Can you work these out from the drawing? Everything is in mm from the part's minimum corner. A direction names the side the tool comes from. Give positions to 0.01 mm unless a question says otherwise; leave off trailing zeros. Loops run counter-clockwise (first coordinate to the right, second up) from the corner with the lowest first, then second, coordinate; pieces in that order, holes last. Notation, with made-up numbers: (-13, 10) - (30, 10) arc R18 cw to (30, 24) - close; hole circle Ø3 at (35, -11.5). An arc over 180 degrees is marked (long way). One line per item, written item: value. Start each with the question number.
Q1. I'm going to push flat-ended pins straight in: P1, Ø1.6, axis at y = 2.5, z = 10, coming from the -X side; P2, Ø1.6, axis at y = 4, z = 10, coming from the +X side; P3, Ø2, axis at y = 2, z = 20.5, coming from the -X side; P4, Ø5, axis at x = 11.44, z = 11.44, coming from the +Y side. Where does each tip first touch, or does it pass through?
Q2. If we mould it in two halves opening along X, with no side actions, what happens to the marked faces 3, 4 and 5? For each: released by +X, released by -X, zero draft, split by the parting line, or undercut.
Q3. I want a section at B-B (z = 9). Please give me the cut outline in (x, y).
Q4. I want a section at A-A (y = 2.2). Please give me the cut outline in (x, z) (1 decimal), then the cut area to 3 significant figures.
Q5. I want a section at D-D (z = 16). Please give me the cut outline in (x, y).
Q6. For the marked faces 1 and 2, which set-ups out of +Z, -Z, +X, -X, +Y, -Y let a thin tool reach every point of the face, with its end or its side?
Q7. I want a section at C-C (x = 9). Please give me the cut outline in (y, z).
Q8. If I drill on line 1 (Y direction, x = 18.25, z = 8); line 2 (X direction, y = 3.25, z = 11) (1 decimal); line 3 (Z direction, x = 7, y = 4) (1 decimal), over which ranges is the centre line in solid material (lowest first)? Write a range as from..to.
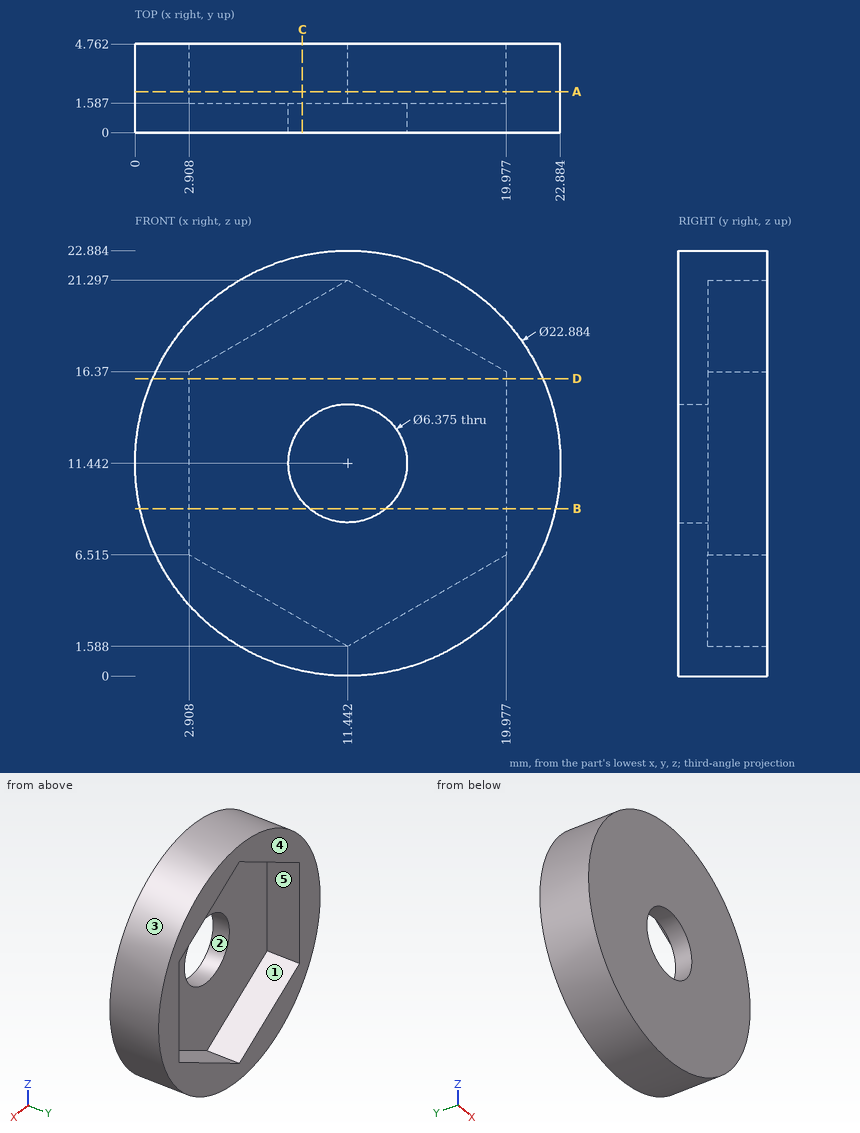
Worked answers:
1. P1: stops at x = 0.02
1. P2: stops at x = 22.87
1. P3: stops at x = 3.32
1. P4: passes through
2. face 3: split by the parting line
2. face 4: zero draft
2. face 5: undercut
3. outline: (0.26, 0) - (9.39, 0) - (9.39, 1.59) - (2.91, 1.59) - (2.91, 4.76) - (0.26, 4.76) - close; (13.49, 0) - (22.62, 0) - (22.62, 4.76) - (19.98, 4.76) - (19.98, 1.59) - (13.49, 1.59) - close
4. outline: circle Ø22.9 at (11.4, 11.4); hole (2.9, 6.5) - (11.4, 1.6) - (20, 6.5) - (20, 16.4) - (11.4, 21.3) - (2.9, 16.4) - close
4. area: 159 mm²
5. outline: (0.95, 0) - (21.94, 0) - (21.94, 4.76) - (19.98, 4.76) - (19.98, 1.59) - (2.91, 1.59) - (2.91, 4.76) - (0.95, 4.76) - close
6. face 1: +Y
6. face 2: +Y, -Y
7. outline: (0, 0.26) - (4.76, 0.26) - (4.76, 3) - (1.59, 3) - (1.59, 9.39) - (0, 9.39) - close; (0, 13.49) - (1.59, 13.49) - (1.59, 19.89) - (4.76, 19.89) - (4.76, 22.62) - (0, 22.62) - close
8. line 1: y = 0..1.59
8. line 2: x = 0..2.9, 20..22.9
8. line 3: z = 0.9..4.2, 18.7..22
